The listing builds one solid part. Answer for the finished solid, in the listing's coordinates (mm). A direction names the side the tool comes from. Give positions to 0.01 mm unless a question says otherwise; leave off trailing zeros. Write each loop counter-clockwise with the first axis right and the second up, starting at its lowest first coordinate (ties: lowest second). Pieces come first, ordered by that corner, then holes. Notation, with made-up numbers: (70.25, -38) -> (122.25, -38) arc R10 cw to (122.25, -26) -> close; hole circle Ø9 at (-23.75, -40). An arc over 180 degrees is marked (long way). Use CSV: the item, a comma, the result in double quotes. Start each with the question number.
from build123d import *

# Parameters (mm, degrees)
F0_R     = 11.125
F1_DEPTH = 7


with BuildPart() as f1:
    # F0 (on Front) → F1 (new body)
    with BuildSketch(Plane.XZ):
        with BuildLine():
            Line((7.176464, 36.03), (-7.176464, 36.00459))
            Line((-7.176464, 36.00459), (-18.705031, 23.047823))
            Line((-18.705031, 23.047823), (-8.872226, 13.929126))
            ThreePointArc((-8.872226, 13.929126), (-8.233094, 12.40237), (-8.963077, 10.916908))
            ThreePointArc((-8.963077, 10.916908), (-9.987883, 9.987883), (-10.916908, 8.963077))
            ThreePointArc((-10.916908, 8.963077), (-12.104836, 8.264456), (-13.462665, 8.500134))
            Line((-13.462665, 8.500134), (-23.6, 14.352928))
            Line((-23.6, 14.352928), (-36.404543, 6.874131))
            Line((-36.404543, 6.874131), (-36.03, -7.176464))
            Line((-36.03, -7.176464), (-22.824744, -18.912232))
            Line((-22.824744, -18.912232), (-13.959667, -8.905918))
            ThreePointArc((-13.959667, -8.905918), (-12.425101, -8.232538), (-10.916908, -8.963077))
            ThreePointArc((-10.916908, -8.963077), (-9.987883, -9.987883), (-8.963077, -10.916908))
            ThreePointArc((-8.963077, -10.916908), (-8.264456, -12.104836), (-8.500134, -13.462665))
            Line((-8.500134, -13.462665), (-14.352928, -23.6))
            Line((-14.352928, -23.6), (-7.413959, -36.001418))
            Line((-7.413959, -36.001418), (7.176464, -36.03))
            Line((7.176464, -36.03), (18.982723, -24.100019))
            Line((18.982723, -24.100019), (8.813928, -13.872823))
            ThreePointArc((8.813928, -13.872823), (8.234726, -12.361877), (8.963077, -10.916908))
            ThreePointArc((8.963077, -10.916908), (9.987883, -9.987883), (10.916908, -8.963077))
            ThreePointArc((10.916908, -8.963077), (12.104836, -8.264456), (13.462665, -8.500134))
            Line((13.462665, -8.500134), (23.6, -14.352928))
            Line((23.6, -14.352928), (36.071911, -7.315997))
            Line((36.071911, -7.315997), (36.03, 7.176464))
            Line((36.03, 7.176464), (24.017932, 19.385856))
            Line((24.017932, 19.385856), (13.90576, 8.847456))
            ThreePointArc((13.90576, 8.847456), (12.385354, 8.23368), (10.916908, 8.963077))
            ThreePointArc((10.916908, 8.963077), (9.987883, 9.987883), (8.963077, 10.916908))
            ThreePointArc((8.963077, 10.916908), (8.26625, 12.095108), (8.490328, 13.445484))
            Line((8.490328, 13.445484), (14.252684, 23.658151))
            Line((14.252684, 23.658151), (7.176464, 36.03))
        make_face()
        Polygon((5.444413, -33.03), (-5.444413, -33.03), (-10.888826, -23.6), (-5.444413, -14.17), (5.444413, -14.17), (10.888826, -23.6), align=None, mode=Mode.SUBTRACT)
        Polygon((-33.03, -5.444413), (-33.03, 5.444413), (-23.6, 10.888826), (-14.17, 5.444413), (-14.17, -5.444413), (-23.6, -10.888826), align=None, mode=Mode.SUBTRACT)
        Circle(F0_R, mode=Mode.SUBTRACT)
        Polygon((33.03, 5.444413), (33.03, -5.444413), (23.6, -10.888826), (14.17, -5.444413), (14.17, 5.444413), (23.6, 10.888826), align=None, mode=Mode.SUBTRACT)
        Polygon((-10.888826, 23.6), (-5.444413, 33.03), (5.444413, 33.03), (10.888826, 23.6), (6.300824, 14.207265), (-5.444413, 14.17), align=None, mode=Mode.SUBTRACT)
    extrude(amount=F1_DEPTH)


solid = f1.part
Q1. Flat-ended cylindrical pins translate along their axes: pin 1 Ø2 at (y, z) = (-3, 2) entering from -X; pin 2 Ø2 at (y, z) = (-4.5, -27) entering from +X; pin 3 Ø3.5 at (y, z) = (-4.5, 1) entering from +X. Find the tip coordinate at first contact, or state that the pin passes through.
Q2. Straight lines are drawn through the part: L1, parallel to Z at x = 0, y = -5 (3 decimals); L2, parallel to X at y = -6, z = 12; L3, parallel to X at y = -3.5, z = 4.5. For each, find the intervals that lie inside material, in ascending order.
Q3. Section D-D on z = 0 is taken. Give the vertices of the cut face in (x, y) (3 decimals).
Q4. Section C-C on x = -21.5 is taken. Give the vertices of the cut face in (y, z).
Q5. The mould has two halves that part along Z. Classify faces 1 (the face through (12.409, -3.451, 8.233)), 2 (the face through (12.997, -3.451, -30.149)), 3 (the face through (-12.86, -3.451, 29.617)): +Z half, -Z half, draft (parallel to the pull), parting line (faces both ways), or undercut.
Q6. Section B-B on z = -27 is taken. Give the vertices of the cut face in (x, y), then the cut area to 3 significant figures.
Q7. Section A-A on x = -2 is taken. Give the vertices of the cut face in (y, z).
Q8. For faces 4 (the face through (9.974, -3.451, -10.002)), 5 (the face through (29.749, -3.451, -10.884)), determine the directions among +Z, -Z, +X, -X, +Y, -Y from which every point of the face is accessible in a straight line to the end or side of a thin tool.
Output:
1,pin 1,"x = -36.3"
1,pin 2,"x = 17.1"
1,pin 3,"x = 36.05"
2,L1,"-36.016 to -33.03, -14.17 to -11.125, 11.125 to 14.187, 33.03 to 36.017"
2,L2,"-27.63 to -19.52, -8.29 to 8.29, 16.93 to 31.28"
2,L3,"-36.34 to -33.03, -14.17 to -10.17, 10.17 to 14.17, 33.03 to 36.04"
3,outline,"(-36.221, -7) -> (-33.03, -7) -> (-33.03, 0) -> (-36.221, 0) -> close; (-14.17, -7) -> (-11.125, -7) -> (-11.125, 0) -> (-14.17, 0) -> close; (11.125, -7) -> (14.17, -7) -> (14.17, 0) -> (11.125, 0) -> close; (33.03, -7) -> (36.051, -7) -> (36.051, 0) -> (33.03, 0) -> close"
4,outline,"(-7, -17.42) -> (0, -17.42) -> (0, -9.68) -> (-7, -9.68) -> close; (-7, 9.68) -> (0, 9.68) -> (0, 13.14) -> (-7, 13.14) -> close"
5,face 1,"undercut"
5,face 2,"-Z half"
5,face 3,"+Z half"
6,outline,"(-12.45, -7) -> (-8.93, -7) -> (-8.93, 0) -> (-12.45, 0) -> close; (8.93, -7) -> (16.11, -7) -> (16.11, 0) -> (8.93, 0) -> close"
6,area,"75.0 mm²"
7,outline,"(-7, -36.01) -> (0, -36.01) -> (0, -33.03) -> (-7, -33.03) -> close; (-7, -14.17) -> (0, -14.17) -> (0, -10.94) -> (-7, -10.94) -> close; (-7, 10.94) -> (0, 10.94) -> (0, 14.18) -> (-7, 14.18) -> close; (-7, 33.03) -> (0, 33.03) -> (0, 36.01) -> (-7, 36.01) -> close"
8,face 4,"+Y, -Y"
8,face 5,"-Z, +X, +Y, -Y"
